Here's how the part is built. I have some questions about the finished solid (model axes, mm). Coordinates: 2 decimals unless noted, no trailing zeros. Write each loop counter-clockwise with the first axis right and the second up, starting at its lowest first coordinate (ties: lowest second). Pieces come first, ordered by that corner, then holes.
Item 1: I want a section at A-A (x = 16.5). Please give me the cut outline in (y, z), and give its area (3 significant figures).
Item 2: Please list where these lines run through material, in increasing order: line 1 (Y direction, x = 11, z = -0.1); line 2 (Z direction, x = 3.75, y = 0.75); line 3 (Z direction, x = 3, y = -1.15).
Item 3: If we mould it in two halves opening along Z, with no side actions, what happens to faces 1 (the face through (1.89, 0.03, -0.05)), 2 (the face through (19.05, 0, 0)), 3 (the face through (10.09, -0.31, 1.39))? For each: pulls with the +Z half, pulls with the -Z half, needs draft (parallel to the pull), parting line crosses it, or undercut.
Item 4: I'm going to push flat-ended pins straight in: P1, Ø2, axis at x = 17, y = 1.5, coming from the -Z side; P2, Ø1.5, axis at x = 16, y = 1, coming from the -Z side. Where does each tip first touch, or does it pass through?
Autodesk Inventor part; units mm, degrees
ref_plane "Work Plane1" through (66.6877, 0, 0) normal (0, 0, -1) x (1, 0, 0)
ref_plane "YZ Plane" through (0, 0, 0) normal (1, 0, 0) x (0, 1, 0)
ref_plane "XZ Plane" through (0, 0, 0) normal (0, 1, 0) x (-1, 0, 0)
sketch "Szkic1" plane through (0, 0, 0) normal (0, 0, 1) x (1, 0, 0)
  line L0 (19.05, 0) -> (19.05, 1.4224)
  line L1 (19.05, 1.4224) -> (2.1082, 1.4224)
  line L2 (0, 2.7686) -> (0, 0.9144)
  line L3 (0, 0.9144) -> (1.397, 0.9144)
  line L4 (1.397, 0.9144) -> (1.9249, 0)
  line L5 (1.9249, 0) -> (19.05, 0)
  line L6 (0, 2.7686) -> (0.5596, 2.7686)
  line L7 (0.5596, 2.7686) -> (2.1082, 1.4224)
  line L8 (-3.81, 0) -> (22.86, 0)
  line L9 (0, -0.5537) -> (0, 3.3223)
  dimension "d0" = 19.05
  dimension "d1" = 1.397
  dimension "d2" = 2.8448
  dimension "d3" = 2.1082
  dimension "d4" = 41
  dimension "d5" = 1.8288
  dimension "d6" = 60
  dimension "d7" = 5.5372
revolve "Bryła" add sketch "Szkic1" angle 360 about axis through (1.9249, 0, 0) along (1, 0, 0) contours L5 L4 L3 L2 L6 L7 L1 L0
sketch "Szkic2" plane through (0, 0, 0) normal (-1, 0, 0) x (0, 0, 1)
  circle A0 centre (0, 0) radius 2.7686
  circle A1 centre (0, 0) radius 0.9144
  line L0 (0.7066, 0.1893) -> (0.8832, 0.2367)
  line L1 (0.7066, -0.1893) -> (0.8832, -0.2367)
  arc A2 (0.7066, -0.1893) -> (0.7066, 0.1893) centre (0, 0) ccw
  arc A3 (0.8832, -0.2367) -> (0.8832, 0.2367) centre (0, 0) ccw
  line L2 (0, -3.876) -> (0, 3.876)
  line L3 (-3.876, 0) -> (3.876, 0)
  line L4 (0.7066, 0.1893) -> (0, 0) construction
  line L5 (0, 0) -> (0.7066, -0.1893) construction
  line L6 (0.1893, 0.7066) -> (0.2367, 0.8832)
  line L7 (0.5173, 0.5173) -> (0.6466, 0.6466)
  arc A4 (0.5173, 0.5173) -> (0.1893, 0.7066) centre (0, 0) ccw
  arc A5 (0.6466, 0.6466) -> (0.2367, 0.8832) centre (0, 0) ccw
  line L8 (-0.5173, 0.5173) -> (-0.6466, 0.6466)
  line L9 (-0.1893, 0.7066) -> (-0.2367, 0.8832)
  arc A6 (-0.1893, 0.7066) -> (-0.5173, 0.5173) centre (0, 0) ccw
  arc A7 (-0.2367, 0.8832) -> (-0.6466, 0.6466) centre (0, 0) ccw
  line L10 (-0.7066, -0.1893) -> (-0.8832, -0.2367)
  line L11 (-0.7066, 0.1893) -> (-0.8832, 0.2367)
  arc A8 (-0.7066, 0.1893) -> (-0.7066, -0.1893) centre (0, 0) ccw
  arc A9 (-0.8832, 0.2367) -> (-0.8832, -0.2367) centre (0, 0) ccw
  line L12 (-0.1893, -0.7066) -> (-0.2367, -0.8832)
  line L13 (-0.5173, -0.5173) -> (-0.6466, -0.6466)
  arc A10 (-0.5173, -0.5173) -> (-0.1893, -0.7066) centre (0, 0) ccw
  arc A11 (-0.6466, -0.6466) -> (-0.2367, -0.8832) centre (0, 0) ccw
  line L14 (0.5173, -0.5173) -> (0.6466, -0.6466)
  line L15 (0.1893, -0.7066) -> (0.2367, -0.8832)
  arc A12 (0.1893, -0.7066) -> (0.5173, -0.5173) centre (0, 0) ccw
  arc A13 (0.2367, -0.8832) -> (0.6466, -0.6466) centre (0, 0) ccw
  dimension "d8" = 1.463
  dimension "d9" = 1.8288
  dimension "d10" = 15
  dimension "d11" = 15
  dimension "d22" = 360
extrude "Szczelina" add sketch "Szkic2" against normal up to next contours L3 A2 L0 A1 | A1 L1 A2 L3 | L3 A8 L10 A1 | A1 L11 A8 L3 | A1 L7 A4 L6 | L9 A6 L8 A1 | A1 L13 A10 L12 | L15 A12 L14 A1
thread "Gwint"
chamfer "Faza1" distance 0.3785 distance2 0.7569 1 edges at (19.05, -1.4224, 0) measured on face at (19.05, 0.5253, 0.4213)
ref_plane "Work Plane1" through (66.6877, 0, 0) normal (0, 0, -1) x (1, 0, 0)
equation "\"d0\" = NLG"
equation "\"d1\" = INTI"
equation "\"d2\" = GD"
equation "\"d3\" = KOH"
equation "\"d4\" = 0.5 * SEWI"
equation "\"d5\" = SW"
equation "\"d7\" = KOD"
equation "\"d8\" = 0.8 * SW"
equation "\"d9\" = SW"
equation "\"d15\" = GEL"
equation "\"d17\" = -0.5 * SPD + 0.5 * GD"
equation "\"d18\" = GUL"
equation "\"NLG\" = 19.05"
equation "\"SW\" = 1.8288"
equation "\"INTI\" = 1.397"
equation "\"GEL\" = 15.3543"
equation "\"KOH\" = 2.1082"
equation "\"KOD\" = 5.5372"
equation "\"GUL\" = 0.75692"
equation "\"SPD\" = 2.08788"
equation "\"GD\" = NND"
equation "\"SEWI\" = 82deg"
equation "\"TOA\" = 30deg"
equation "\"GD1\" = SPD"
equation "\"EPV\" = 3.74448"
equation "\"THREADDIA\" = 2.8448"
equation "\"BDM\" = NND"
equation "\"NND\" = 2.8448"
equation "\"GAL\" = 1.5875"
equation "\"E0\" = 1.155 * SW"
properties part number "ANSI B18.3 - 4-40 UNC x 0,75" material "Stal, miękka"
Answer:
1. outline: circle Ø2.84 at (0, 0)
1. area: 6.36 mm2
2. line 1: y = -1.42 to 1.42
2. line 2: z = -1.21 to 1.21
2. line 3: z = -0.84 to 0.84
3. face 1: undercut
3. face 2: needs draft
3. face 3: parting line crosses it
4. P1: stops at z = -1.33
4. P2: stops at z = -1.4
